from build123d import *

# Parameters (mm, degrees)
CROQUIS1_W              = 5.9
CROQUIS1_H              = 12.5
CROQUIS1_W_2            = 5.3
CROQUIS1_H_2            = 10
CROQUIS1_W_3            = 5.7277
CROQUIS1_H_3            = 7.4295
SALIENTE_EXTRUIR1_DEPTH = 1
CROQUIS2_W              = 5.9
CROQUIS2_H              = 12.5
CROQUIS2_W_2            = 5.3
CROQUIS2_H_2            = 10
CROQUIS2_W_3            = 5.7277
CROQUIS2_H_3            = 7.4295
SALIENTE_EXTRUIR2_DEPTH = 7
CROQUIS3_W              = 1.2
CROQUIS3_H              = 7.4295
CROQUIS3_H_2            = 10
CROQUIS3_H_3            = 12.5
SALIENTE_EXTRUIR3_DEPTH = 1.5
CHAFL_N1_SIZE           = 1
REDONDEO1_R             = 2


with BuildPart() as part:
    # Croquis1 → Saliente-Extruir1 (new body)
    with BuildSketch(Plane.XY):
        with BuildLine():
            Line((6.325110646, 1.27705094), (31.213497595, 1.27705094))
            ThreePointArc((31.213497595, 1.27705094), (33.334817939, 2.155730596), (34.213497595, 4.27705094))
            Line((34.213497595, 4.27705094), (34.213497595, 46.12294906))
            ThreePointArc((34.213497595, 46.12294906), (33.334817939, 48.244269404), (31.213497595, 49.12294906))
            Line((31.213497595, 49.12294906), (6.325110646, 49.12294906))
            Line((6.325110646, 49.12294906), (6.325110646, 35.928313067))
            Line((6.325110646, 35.928313067), (7.004112389, 35.928313067))
            Line((7.004112389, 35.928313067), (7.004112389, 14.471686933))
            Line((7.004112389, 14.471686933), (6.325110646, 14.471686933))
            Line((6.325110646, 14.471686933), (6.325110646, 1.27705094))
        make_face()
        with Locations((27.45822767, 37.510466453)):
            Rectangle(CROQUIS1_W, CROQUIS1_H, mode=Mode.SUBTRACT)
        with Locations((27.75822767, 22.260466453)):
            Rectangle(CROQUIS1_W_2, CROQUIS1_H_2, mode=Mode.SUBTRACT)
        with Locations((27.54437767, 9.545716453)):
            Rectangle(CROQUIS1_W_3, CROQUIS1_H_3, mode=Mode.SUBTRACT)
        with Locations((19.05822767, 37.510466453)):
            Rectangle(CROQUIS1_W, CROQUIS1_H, mode=Mode.SUBTRACT)
        with Locations((19.35822767, 22.260466453)):
            Rectangle(CROQUIS1_W_2, CROQUIS1_H_2, mode=Mode.SUBTRACT)
        with Locations((19.14437767, 9.545716453)):
            Rectangle(CROQUIS1_W_3, CROQUIS1_H_3, mode=Mode.SUBTRACT)
        with Locations((10.65822767, 37.510466453)):
            Rectangle(CROQUIS1_W, CROQUIS1_H, mode=Mode.SUBTRACT)
        with Locations((10.95822767, 22.260466453)):
            Rectangle(CROQUIS1_W_2, CROQUIS1_H_2, mode=Mode.SUBTRACT)
        with Locations((10.74437767, 9.545716453)):
            Rectangle(CROQUIS1_W_3, CROQUIS1_H_3, mode=Mode.SUBTRACT)
    extrude(amount=-SALIENTE_EXTRUIR1_DEPTH)

    # Croquis2 → Saliente-Extruir2 (add)
    with BuildSketch(Plane.XY):
        Polygon((36.213497595, 53.820046244), (1.576275643, 53.820046244), (1.576275643, 35.928313067), (3.319198905, 35.928313067), (3.319198905, 14.471686933), (1.576275643, 14.471686933), (1.576275643, -3.420839566), (36.213497595, -3.420839566), align=None)
        with Locations((27.45822767, 37.510466453)):
            Rectangle(CROQUIS2_W, CROQUIS2_H, mode=Mode.SUBTRACT)
        with Locations((27.75822767, 22.260466453)):
            Rectangle(CROQUIS2_W_2, CROQUIS2_H_2, mode=Mode.SUBTRACT)
        with Locations((27.54437767, 9.545716453)):
            Rectangle(CROQUIS2_W_3, CROQUIS2_H_3, mode=Mode.SUBTRACT)
        with Locations((19.14437767, 9.545716453)):
            Rectangle(CROQUIS2_W_3, CROQUIS2_H_3, mode=Mode.SUBTRACT)
        with Locations((19.35822767, 22.260466453)):
            Rectangle(CROQUIS2_W_2, CROQUIS2_H_2, mode=Mode.SUBTRACT)
        with Locations((19.05822767, 37.510466453)):
            Rectangle(CROQUIS2_W, CROQUIS2_H, mode=Mode.SUBTRACT)
        with Locations((10.65822767, 37.510466453)):
            Rectangle(CROQUIS2_W, CROQUIS2_H, mode=Mode.SUBTRACT)
        with Locations((10.95822767, 22.260466453)):
            Rectangle(CROQUIS2_W_2, CROQUIS2_H_2, mode=Mode.SUBTRACT)
        with Locations((10.74437767, 9.545716453)):
            Rectangle(CROQUIS2_W_3, CROQUIS2_H_3, mode=Mode.SUBTRACT)
    extrude(amount=SALIENTE_EXTRUIR2_DEPTH)

    # Croquis3 → Saliente-Extruir3 (add)
    with BuildSketch(Plane(origin=(0, 0, -1), x_dir=(-1, 0, 0), z_dir=(0, 0, -1))):
        with Locations((-29.80822767, 9.545716453)):
            Rectangle(CROQUIS3_W, CROQUIS3_H)
        with Locations((-21.40822767, 9.545716453)):
            Rectangle(CROQUIS3_W, CROQUIS3_H)
        with Locations((-25.28052767, 9.545716453)):
            Rectangle(CROQUIS3_W, CROQUIS3_H)
        with Locations((-16.88052767, 9.545716453)):
            Rectangle(CROQUIS3_W, CROQUIS3_H)
        with Locations((-13.00822767, 9.545716453)):
            Rectangle(CROQUIS3_W, CROQUIS3_H)
        with Locations((-8.48052767, 9.545716453)):
            Rectangle(CROQUIS3_W, CROQUIS3_H)
        with Locations((-29.80822767, 22.260466453)):
            Rectangle(CROQUIS3_W, CROQUIS3_H_2)
        with Locations((-21.40822767, 22.260466453)):
            Rectangle(CROQUIS3_W, CROQUIS3_H_2)
        with Locations((-25.70822767, 22.260466453)):
            Rectangle(CROQUIS3_W, CROQUIS3_H_2)
        with Locations((-17.30822767, 22.260466453)):
            Rectangle(CROQUIS3_W, CROQUIS3_H_2)
        with Locations((-13.00822767, 22.260466453)):
            Rectangle(CROQUIS3_W, CROQUIS3_H_2)
        with Locations((-8.90822767, 22.260466453)):
            Rectangle(CROQUIS3_W, CROQUIS3_H_2)
        with Locations((-29.80822767, 37.510466453)):
            Rectangle(CROQUIS3_W, CROQUIS3_H_3)
        with Locations((-25.10822767, 37.510466453)):
            Rectangle(CROQUIS3_W, CROQUIS3_H_3)
        with Locations((-21.40822767, 37.510466453)):
            Rectangle(CROQUIS3_W, CROQUIS3_H_3)
        with Locations((-16.70822767, 37.510466453)):
            Rectangle(CROQUIS3_W, CROQUIS3_H_3)
        with Locations((-13.00822767, 37.510466453)):
            Rectangle(CROQUIS3_W, CROQUIS3_H_3)
        with Locations((-8.30822767, 37.510466453)):
            Rectangle(CROQUIS3_W, CROQUIS3_H_3)
    extrude(amount=-SALIENTE_EXTRUIR3_DEPTH)

    # Chaflán1
    chafl_n1_edges = [part.edges().sort_by_distance(p)[0] for p in [
        (30.40822767, 9.545716453, 0.5),
        (24.68052767, 9.545716453, 0.5),
        (22.00822767, 9.545716453, 0.5),
        (16.28052767, 9.545716453, 0.5),
        (13.60822767, 9.545716453, 0.5),
        (7.88052767, 9.545716453, 0.5),
        (30.40822767, 22.260466453, 0.5),
        (25.10822767, 22.260466453, 0.5),
        (22.00822767, 22.260466453, 0.5),
        (16.70822767, 22.260466453, 0.5),
        (13.60822767, 22.260466453, 0.5),
        (8.30822767, 22.260466453, 0.5),
        (30.40822767, 37.510466453, 0.5),
        (24.50822767, 37.510466453, 0.5),
        (22.00822767, 37.510466453, 0.5),
        (16.10822767, 37.510466453, 0.5),
        (13.60822767, 37.510466453, 0.5),
        (7.70822767, 37.510466453, 0.5),
    ]]
    chamfer(chafl_n1_edges, length=CHAFL_N1_SIZE)

    # Redondeo1
    redondeo1_edges = [part.edges().sort_by_distance(p)[0] for p in [
        (18.894886619, -3.420839566, 7),
        (36.213497595, 25.199603339, 7),
        (18.894886619, 53.820046244, 7),
        (36.213497595, -3.420839566, 3.5),
        (36.213497595, 53.820046244, 3.5),
    ]]
    fillet(redondeo1_edges, radius=REDONDEO1_R)


solid = part.part
Geometry: final body of the model. Coordinates: model frame, mm. A direction names the side the tool comes from. Give positions to 0.01 mm unless a question says otherwise; leave off trailing zeros. Order: outer loops, then holes, each group sorted by start corner. A loop starts at its lowest first (then second) coordinate and runs counter-clockwise, first axis right, second up. Notation, with made-up numbers: (-8.75, 7) -> (32.25, 7) arc R22 cw to (32.25, 26) -> close; hole circle Ø3 at (44.5, 27). An arc over 180 degrees is marked (long way). Write each question's results on one line, items separated by ' | '.
1) Cut plane A-A (x = 20). Output: boundary loops of the cut face in (y, z).
Geometry says:
outline: (-3.42, 0) -> (1.28, 0) -> (1.28, -1) -> (5.83, -1) -> (5.83, 7) -> (-1.42, 7) arc R2 ccw to (-3.42, 5) -> close; (13.26, -1) -> (17.26, -1) -> (17.26, 7) -> (13.26, 7) -> close; (27.26, -1) -> (31.26, -1) -> (31.26, 7) -> (27.26, 7) -> close; (43.76, -1) -> (49.12, -1) -> (49.12, 0) -> (53.82, 0) -> (53.82, 5) arc R2 ccw to (51.82, 7) -> (43.76, 7) -> close
2) Cut plane C-C (z = 2.25). Give the number of separate pieces and of enclosed holes in the cut face, and give its area (3 significant figures).
Geometry says:
separate pieces: 1 | enclosed holes: 9 | area: 1,440 mm²
3) Draft query along X for faces 1 (the face through (18.12, -2.82, 6.43)), 2 (the face through (19, 43.76, 3)), 3 (the face through (36.213, 25, 2)). Return one class per face: released by +X, released by -X, zero draft, split by the parting line, or undercut.
Geometry says:
face 1: zero draft | face 2: undercut | face 3: released by +X
4) Line query: line 1 along X through (y, z) = (25, 2.5); line 2 along X through (y, z) = (10, 3.5); line 3 along Y through (x, z) = (17.5, 1). Output: solid intervals per line, ascending.
Geometry says:
line 1: x = 3.32 to 8.31, 13.61 to 16.71, 22.01 to 25.11, 30.41 to 36.21 | line 2: x = 1.58 to 7.88, 13.61 to 16.28, 22.01 to 24.68, 30.41 to 36.21 | line 3: y = -3.42 to 5.83, 13.26 to 17.26, 27.26 to 31.26, 43.76 to 53.82
5) First-contact query: pin 1 Ø0.5 at (x, z) = (6.5, -0.5) entering from -Y; pin 2 Ø3.5 at (y, z) = (20, 5) entering from -X; pin 3 Ø0.5 at (y, z) = (42.5, -0.5) entering from -X. Flat tips, straight axial feed; report the tip coordinate or a pass-through.
Geometry says:
pin 1: stops at y = 1.28 | pin 2: stops at x = 3.32 | pin 3: stops at x = 6.33
6) Set-up query: faces 4 (the face through (33.31, 2.13, -0.49)), 5 (the face through (16.108, 37, 4)), 6 (the face through (8.908, 37, 0)). Return all of +Z, -Z, +X, -X, +Y, -Y with unobstructed straight access to the full face (end or side cutting, diameter ignored); none if empty.
Geometry says:
face 4: -Z, +X, -Y | face 5: +Z | face 6: +Z, -Z
7) Cut plane B-B (y = 50.5). Output: boundary loops of the cut face in (x, z), and give its area (3 significant figures).
Geometry says:
outline: (1.58, 0) -> (36.21, 0) -> (36.21, 5) arc R2 ccw to (34.21, 7) -> (1.58, 7) -> close | area: 242 mm²
